The listing builds one solid part. Answer for the finished solid, in the listing's coordinates (mm). A direction names the side the tool comes from. Give positions to 0.01 mm unless a question says otherwise; leave off trailing zeros. Loops run counter-clockwise (first coordinate to the right, second up) from the corner with the lowest first, then second, coordinate; pieces in that order, holes last. Notation, with made-up numbers: M 37,65 L 57,65 A18 ccw 57,70 Z; hole C 52,-36 d8. An arc over 180 degrees is marked long. Use one line per item in the form item = value. Start each with the question number.
1. Each of these flat-tipped pins is pushed along its axis until it touches: pin 1 Ø3.5 at (y, z) = (0, 35.5) entering from +X; pin 2 Ø3.5 at (y, z) = (0, 41) entering from -X; pin 3 Ø5 at (x, z) = (26, 1) entering from +Y. Where does it stop, or does it pass through?
2. The part is cut by section C-C (x = -47.5). Write down the section's boundary in (y, z), and give its area (3 significant figures).
3. The part is cut by section A-A (y = 5.75). Write down the section's boundary in (x, z).
4. The part is cut by section B-B (z = -41.25). Write down the section's boundary in (x, y), and give its area (3 significant figures).
5. For faces 5 (the face through (-1, 5, 45.3)), 6 (the face through (-55.197, 0.021, 20.911)), 7 (the face through (-54.909, 0, 38)), 8 (the face through (54.909, 0, -38)), 9 (the face through (55.213, 0.021, 20.966)), determine the directions among +Z, -Z, +X, -X, +Y, -Y from which every point of the face is accessible in a straight line to the end or side of a thin tool.
6. The part is cut by section D-D (x = 27.5). Write down the section's boundary in (y, z).
7. Straight lines are drawn through the part: line 1 (X direction, y = 0.55, z = 41.25); line 2 (X direction, y = 0.75, z = 25); line 3 (Z direction, x = -48, y = 3.75). For each, find the intervals that lie inside material, in ascending order. Write a range as from..to.
8. The mould has two halves that part along Z. Classify faces 1 (the face through (-54.909, 0, 0)), 2 (the face through (52.667, 3.085, 47.087)), 3 (the face through (-55.197, 0.021, -29.089)), 4 (the face through (54.2, 0.02, -24.67)): released by +Z, released by -Z, zero draft, split by the parting line, or undercut.
from build123d import *

# Parameters (mm, degrees)
BOSS_EXTRUDE1_DEPTH   = 7.8
BOSS_EXTRUDE1_2_DEPTH = 7.8
BOSS_EXTRUDE2_DEPTH   = 1.5
SKETCH5_R             = 1.6
CUT_EXTRUDE1_DEPTH    = 74.072152553
SKETCH6_R             = 1.525
CUT_EXTRUDE2_DEPTH    = 74.072152553
SKETCH7_R             = 4.025
SKETCH7_R_2           = 1.525
BOSS_EXTRUDE3_DEPTH   = 1.5
FILLET1_R             = 7
SKETCH8_R             = 2.75
CUT_EXTRUDE3_DEPTH    = 3


with BuildPart() as part:
    # Sketch1 → Boss-Extrude1 (new body)
    with BuildSketch(Plane(origin=(0, 0, 0), x_dir=(1, 0, 0), z_dir=(0, 1, 0))):
        with BuildLine():
            Line((-50.55, -45.3), (50.55, -45.3))
            Line((50.55, -45.3), (53.904101966, -45.3))
            ThreePointArc((53.904101966, -45.3), (52.641650066, -47.10624304), (50.55, -47.8))
            Line((50.55, -47.8), (-50.55, -47.8))
            ThreePointArc((-50.55, -47.8), (-52.641650066, -47.10624304), (-53.904101966, -45.3))
            Line((-53.904101966, -45.3), (-50.55, -45.3))
        make_face()
    extrude(amount=BOSS_EXTRUDE1_DEPTH)



with BuildPart() as body_2:
    # Sketch1 → Boss-Extrude1 2 (new body)
    with BuildSketch(Plane(origin=(0, 0, 0), x_dir=(1, 0, 0), z_dir=(0, 1, 0))):
        with BuildLine():
            Line((-50.55, 45.3), (50.55, 45.3))
            Line((50.55, 45.3), (53.904101966, 45.3))
            ThreePointArc((53.904101966, 45.3), (52.641650066, 47.10624304), (50.55, 47.8))
            Line((50.55, 47.8), (-50.55, 47.8))
            ThreePointArc((-50.55, 47.8), (-52.641650066, 47.10624304), (-53.904101966, 45.3))
            Line((-53.904101966, 45.3), (-50.55, 45.3))
        make_face()
    extrude(amount=BOSS_EXTRUDE1_2_DEPTH)


with BuildPart() as part_1:
    add(part.part)

    add(body_2.part)  # Boss-Extrude2 merges body 2
    # Sketch3 → Boss-Extrude2 (add, symmetric)
    with BuildSketch(Plane(origin=(0, 0, 0), x_dir=(1, 0, 0), z_dir=(0, 1, 0))):
        with BuildLine():
            Line((-50.55, 47.8), (50.55, 47.8))
            ThreePointArc((50.55, 47.8), (52.394661968, 47.27442805), (53.685322458, 45.855555556))
            ThreePointArc((53.685322458, 45.855555556), (54.054082597, 45.450163414), (54.581128874, 45.3))
            Line((54.581128874, 45.3), (54.909101966, 45.3))
            Line((54.909101966, 45.3), (54.909101966, -45.3))
            Line((54.909101966, -45.3), (54.581128874, -45.3))
            ThreePointArc((54.581128874, -45.3), (54.054082597, -45.450163414), (53.685322458, -45.855555556))
            ThreePointArc((53.685322458, -45.855555556), (52.394661968, -47.27442805), (50.55, -47.8))
            Line((50.55, -47.8), (-50.55, -47.8))
            ThreePointArc((-50.55, -47.8), (-52.394661968, -47.27442805), (-53.685322458, -45.855555556))
            ThreePointArc((-53.685322458, -45.855555556), (-54.054082597, -45.450163414), (-54.581128874, -45.3))
            Line((-54.581128874, -45.3), (-54.909101966, -45.3))
            Line((-54.909101966, -45.3), (-54.909101966, 45.3))
            Line((-54.909101966, 45.3), (-54.581128874, 45.3))
            ThreePointArc((-54.581128874, 45.3), (-54.054082597, 45.450163414), (-53.685322458, 45.855555556))
            ThreePointArc((-53.685322458, 45.855555556), (-52.394661968, 47.27442805), (-50.55, 47.8))
        make_face()
    extrude(amount=BOSS_EXTRUDE2_DEPTH, both=True)

    # Sketch5 → Cut-Extrude1 (cut, through all)
    with BuildSketch(Plane(origin=(0, 1.5, 0), x_dir=(1, 0, 0), z_dir=(0, 1, 0))):
        with Locations(Location((-47.5, 41.25, 0), (0, 0, 270))):
            Circle(SKETCH5_R)
        with Locations(Location((47.5, 41.25, 0), (0, 0, 90))):
            Circle(SKETCH5_R)
        with Locations(Location((47.5, -41.25, 0), (0, 0, 270))):
            Circle(SKETCH5_R)
        with Locations(Location((-47.5, -41.25, 0), (0, 0, 90))):
            Circle(SKETCH5_R)
    extrude(amount=-CUT_EXTRUDE1_DEPTH, mode=Mode.SUBTRACT)

    # Sketch6 → Cut-Extrude2 (cut, through all)
    with BuildSketch(Plane(origin=(0, 1.5, 0), x_dir=(1, 0, 0), z_dir=(0, 1, 0))):
        with Locations(Location((-52.709101966, 25, 0), (0, 0, 270))):
            Circle(SKETCH6_R)
        with Locations(Location((52.709101966, 25, 0), (0, 0, 90))):
            Circle(SKETCH6_R)
        with Locations(Location((52.709101966, -25, 0), (0, 0, 270))):
            Circle(SKETCH6_R)
        with Locations(Location((-52.709101966, -25, 0), (0, 0, 90))):
            Circle(SKETCH6_R)
    extrude(amount=-CUT_EXTRUDE2_DEPTH, mode=Mode.SUBTRACT)

    # Sketch7 → Boss-Extrude3 (add, symmetric)
    # profile 1 of 4: a face of its own
    with BuildSketch(Plane(origin=(0, 0, 0), x_dir=(1, 0, 0), z_dir=(0, 1, 0))):
        with Locations((-52.709101966, 25)):
            Circle(SKETCH7_R)
        with Locations(Location((-52.709101966, 25, 0), (0, 0, 270))):
            Circle(SKETCH7_R_2, mode=Mode.SUBTRACT)
    # profile 2 of 4: a face of its own
    with BuildSketch(Plane(origin=(0, 0, 0), x_dir=(1, 0, 0), z_dir=(0, 1, 0))):
        with Locations((-52.709101966, -25)):
            Circle(SKETCH7_R)
        with Locations(Location((-52.709101966, -25, 0), (0, 0, 90))):
            Circle(SKETCH7_R_2, mode=Mode.SUBTRACT)
    # profile 3 of 4: a face of its own
    with BuildSketch(Plane(origin=(0, 0, 0), x_dir=(1, 0, 0), z_dir=(0, 1, 0))):
        with Locations((52.709101966, 25)):
            Circle(SKETCH7_R)
        with Locations(Location((52.709101966, 25, 0), (0, 0, 90))):
            Circle(SKETCH7_R_2, mode=Mode.SUBTRACT)
    # profile 4 of 4: a face of its own
    with BuildSketch(Plane(origin=(0, 0, 0), x_dir=(1, 0, 0), z_dir=(0, 1, 0))):
        with Locations((52.709101966, -25)):
            Circle(SKETCH7_R)
        with Locations(Location((52.709101966, -25, 0), (0, 0, 270))):
            Circle(SKETCH7_R_2, mode=Mode.SUBTRACT)
    extrude(amount=BOSS_EXTRUDE3_DEPTH, both=True)

    # Fillet1
    fillet1_edges = [part_1.edges().sort_by_distance(p)[0] for p in [
        (-54.909101966, 0, 28.370552625),
        (-54.909101966, 0, 21.629447375),
        (54.909101966, 0, -28.370552625),
        (54.909101966, 0, -21.629447375),
        (54.909101966, 0, 21.629447375),
        (54.909101966, 0, 28.370552625),
        (-54.909101966, 0, -21.629447375),
        (-54.909101966, 0, -28.370552625),
    ]]
    fillet(fillet1_edges, radius=FILLET1_R)

    # Sketch8 → Cut-Extrude3 (cut)
    with BuildSketch(Plane(origin=(0, 1.5, 0), x_dir=(1, 0, 0), z_dir=(0, 1, 0))):
        with Locations(Location((-47.5, -41.25, 0), (0, 0, 270))):
            Circle(SKETCH8_R)
        with Locations(Location((-47.5, 41.25, 0), (0, 0, 90))):
            Circle(SKETCH8_R)
        with Locations(Location((47.5, 41.25, 0), (0, 0, 270))):
            Circle(SKETCH8_R)
        with Locations(Location((47.5, -41.25, 0), (0, 0, 90))):
            Circle(SKETCH8_R)
    extrude(amount=-CUT_EXTRUDE3_DEPTH, mode=Mode.SUBTRACT)


solid = part_1.part
Derived:
q1.pin_1 = 54.91
q1.pin_2 = -54.91
q1.pin_3 = 1.5
q2.outline = M -1.5,-47.8 L 7.8,-47.8 L 7.8,-45.3 L 1.5,-45.3 L 1.5,-44 L -1.5,-44 Z; M -1.5,-38.5 L 1.5,-38.5 L 1.5,38.5 L -1.5,38.5 Z; M -1.5,44 L 1.5,44 L 1.5,45.3 L 7.8,45.3 L 7.8,47.8 L -1.5,47.8 Z
q2.area = 285 mm2
q3.outline = M -53.9,-45.3 A3.5 ccw -50.55,-47.8 L 50.55,-47.8 A3.5 ccw 53.9,-45.3 Z; M -53.9,45.3 L 53.9,45.3 A3.5 ccw 50.55,47.8 L -50.55,47.8 A3.5 ccw Z
q4.outline = M -54.91,-1.5 L -50.25,-1.5 L -50.25,1.5 L -54.91,1.5 Z; M -44.75,-1.5 L 44.75,-1.5 L 44.75,1.5 L -44.75,1.5 Z; M 50.25,-1.5 L 54.91,-1.5 L 54.91,1.5 L 50.25,1.5 Z
q4.area = 296 mm2
q5.face_5 = +X, -X, +Y
q5.face_6 = -X, +Y, -Y
q5.face_7 = +Z, -X, +Y, -Y
q5.face_8 = -Z, +X, +Y, -Y
q5.face_9 = +X, +Y, -Y
q6.outline = M -1.5,-47.8 L 7.8,-47.8 L 7.8,-45.3 L 1.5,-45.3 L 1.5,45.3 L 7.8,45.3 L 7.8,47.8 L -1.5,47.8 Z
q7.line_1 = -54.91..-50.25, -44.75..44.75, 50.25..54.91
q7.line_2 = -56.73..-54.23, -51.18..51.18, 54.23..56.73
q7.line_3 = -47.8..-45.3, 45.3..47.8
q8.face_1 = undercut
q8.face_2 = released by +Z
q8.face_3 = released by -Z
q8.face_4 = undercut
